from build123d import *

# Parameters (mm, degrees)
SKETCH1_R           = 2.2
SKETCH1_W           = 25.4
SKETCH1_H           = 25.4
SKETCH1_W_2         = 4.6228
SKETCH1_H_2         = 4.6228
SKETCH1_W_3         = 12.7
SKETCH1_H_3         = 12.7
BOSS_EXTRUDE1_DEPTH = 12.7
BOSS_EXTRUDE2_START = 12.7
SKETCH1_3_W         = 4.6228
SKETCH1_3_H         = 4.6228
BOSS_EXTRUDE2_DEPTH = 1.6
FILLET1_R           = 6.35
FILLET2_R           = 0.6
FILLET3_R           = 1


with BuildPart() as part:
    # Sketch1 → Boss-Extrude1 (new body)
    # profile 1 of 5: a face of its own
    with BuildSketch(Plane.XY):
        Polygon((6.35, -31.75), (0, -25.4), (25.4, -25.4), (25.4, 0), (31.75, -6.35), (44.45, -6.35), (44.45, -19.05), (76.2, -19.05), (76.2, -31.75), align=None)
        with Locations((38.1, -12.7)):
            Circle(SKETCH1_R, mode=Mode.SUBTRACT)
    # profile 2 of 5: a face of its own
    with BuildSketch(Plane.XY):
        with Locations((12.7, -12.7)):
            Rectangle(SKETCH1_W, SKETCH1_H)
        with Locations((19.05, -19.05)):
            Circle(SKETCH1_R, mode=Mode.SUBTRACT)
        with Locations((19.05, -6.35)):
            Circle(SKETCH1_R, mode=Mode.SUBTRACT)
        with Locations((6.35, -6.35)):
            Rectangle(SKETCH1_W_2, SKETCH1_H_2, mode=Mode.SUBTRACT)
        with Locations((6.35, -19.05)):
            Rectangle(SKETCH1_W_2, SKETCH1_H_2, mode=Mode.SUBTRACT)
    # profile 3 of 5: a face of its own
    with BuildSketch(Plane.XY):
        with Locations((6.35, -19.05)):
            Rectangle(SKETCH1_W_2, SKETCH1_H_2)
    # profile 4 of 5: a face of its own
    with BuildSketch(Plane.XY):
        with Locations((6.35, -6.35)):
            Rectangle(SKETCH1_W_2, SKETCH1_H_2)
    # profile 5 of 5: a face of its own
    with BuildSketch(Plane.XY):
        with Locations((82.55, -25.4)):
            Rectangle(SKETCH1_W_3, SKETCH1_H_3)
    extrude(amount=BOSS_EXTRUDE1_DEPTH)

    # Sketch1<3> → Boss-Extrude2 (add)
    with BuildSketch(Plane.XY.offset(BOSS_EXTRUDE2_START)):
        with Locations((6.35, -6.35)):
            Rectangle(SKETCH1_3_W, SKETCH1_3_H)
        with Locations((6.35, -19.05)):
            Rectangle(SKETCH1_3_W, SKETCH1_3_H)
    extrude(amount=BOSS_EXTRUDE2_DEPTH)

    # Fillet1
    fillet1_edges = [part.edges().sort_by_distance(p)[0] for p in [
        (88.9, -31.75, 6.35),
        (88.9, -19.05, 6.35),
        (44.45, -19.05, 6.35),
        (44.45, -6.35, 6.35),
        (31.75, -6.35, 6.35),
        (25.4, 0, 6.35),
        (6.35, -31.75, 6.35),
        (0, -25.4, 6.35),
        (0, 0, 6.35),
    ]]
    fillet(fillet1_edges, radius=FILLET1_R - 0.0001)  # a hair under: the kernel refuses the full size

    # Fillet2
    fillet2_edges = [part.edges().sort_by_distance(p)[0] for p in [
        (6.35, -8.6614, 14.3),
        (4.0386, -8.6614, 13.5),
        (8.6614, -8.6614, 13.5),
        (8.6614, -4.0386, 13.5),
        (4.0386, -6.35, 14.3),
        (4.0386, -4.0386, 13.5),
        (8.6614, -6.35, 14.3),
        (6.35, -4.0386, 14.3),
        (6.35, -21.3614, 14.3),
        (4.0386, -21.3614, 13.5),
        (8.6614, -21.3614, 13.5),
        (8.6614, -16.7386, 13.5),
        (4.0386, -19.05, 14.3),
        (4.0386, -16.7386, 13.5),
        (8.6614, -19.05, 14.3),
        (6.35, -16.7386, 14.3),
    ]]
    fillet(fillet2_edges, radius=FILLET2_R)

    # Fillet3
    fillet3_edges = [part.edges().sort_by_distance(p)[0] for p in [
        (3.175, -28.575, 0),
        (0, -14.55984265, 0),
        (14.55984265, 0, 0),
        (28.575, -3.175, 0),
        (36.24015735, -6.35, 0),
        (66.675, -19.05, 0),
        (45.76515735, -31.75, 0),
        (1.85984265, -1.85984265, 0),
        (0.483357357, -25.199786827, 0),
        (6.550213173, -31.266642643, 0),
        (25.199786827, -0.483357357, 0),
        (42.59015735, -8.20984265, 0),
        (87.04015735, -20.90984265, 0),
        (87.04015735, -29.89015735, 0),
        (45.76515735, -31.75, 12.7),
        (3.175, -28.575, 12.7),
        (66.675, -19.05, 12.7),
        (36.24015735, -6.35, 12.7),
        (28.575, -3.175, 12.7),
        (14.55984265, 0, 12.7),
        (0, -14.55984265, 12.7),
        (1.85984265, -1.85984265, 12.7),
        (0.483357357, -25.199786827, 12.7),
        (6.550213173, -31.266642643, 12.7),
        (25.199786827, -0.483357357, 12.7),
        (42.59015735, -8.20984265, 12.7),
        (87.04015735, -20.90984265, 12.7),
        (87.04015735, -29.89015735, 12.7),
        (46.30984265, -17.19015735, 0),
        (46.30984265, -17.19015735, 12.7),
        (31.950213173, -5.866642643, 0),
        (31.950213173, -5.866642643, 12.7),
    ]]
    fillet(fillet3_edges, radius=FILLET3_R)


solid = part.part
The listing builds one solid part. Answer for the finished solid, in the listing's coordinates (mm). A direction names the side the tool comes from. Give positions to 0.01 mm unless a question says otherwise; leave off trailing zeros. Write each loop counter-clockwise with the first axis right and the second up, starting at its lowest first coordinate (ties: lowest second). Pieces come first, ordered by that corner, then holes.
1) A tool of negligible diameter and unlimited length cuts with its end or side. For faces 4 (the face through (28.381, -3.406, 12.415)), 5 (the face through (66, -19.05, 6)), from which of +Z, -Z, +X, -X, +Y, -Y can it reach the whole face along a straight path? Write none if from no direction.
2) For a pull along Y with two mould halves and no side action, classify faces 1 (the face through (17.304, -20.389, 6.261)), 2 (the face through (1.91, -1.81, 6.42)), 3 (the face through (3.369, -28.344, 12.415)) as pulls with the +Y half, pulls with the -Y half, needs draft (parallel to the pull), parting line crosses it, or undercut.
3) Find the intervals of material crossed by L1, parallel to Y at x = 19.05, z = 4.5; L2, parallel to Y at x = 81.5, z = 3; L3, parallel to Z at x = 62, y = -26, in increasing order.
4) Given P1, Ø2, axis at x = 65, z = 5.5, coming from the +Y side; P2, Ø4, axis at x = 38.1, y = -12.7, coming from the -Z side; P3, Ø5, axis at x = 37, z = 9, coming from the +Y side; P4, Ø0.8, axis at x = 7, z = 13.5, coming from the +Y side, each flat-ended and moving along its own axis, determine where each tip first touches the part or whether it passes through.
5) Section A-A (z = 5) is taken. Count the separate pieces of the cut face and the enclosed holes in it, and give its area (3 significant figures).
6) Section C-C (x = 56.5) is taken. Write down the section's boundary in (y, z), and give its area (3 significant figures).
7) Section B-B (x = 19.05) is taken. Write down the section's boundary in (y, z), and give its area (3 significant figures).
Response:
1. face 4: +Z, +X, +Y
1. face 5: +Z, -Z, +X, +Y
2. face 1: undercut
2. face 2: pulls with the +Y half
2. face 3: pulls with the -Y half
3. L1: y = -31.75 to -21.25, -16.85 to -8.55, -4.15 to 0
3. L2: y = -31.75 to -19.05
3. L3: z = 0 to 12.7
4. P1: stops at y = -19.05
4. P2: passes through
4. P3: stops at y = -6.35
4. P4: stops at y = -4.04
5. separate pieces: 1
5. enclosed holes: 3
5. area: 1,780 mm2
6. outline: (-31.75, 1) arc R1 ccw to (-30.75, 0) - (-20.05, 0) arc R1 ccw to (-19.05, 1) - (-19.05, 11.7) arc R1 ccw to (-20.05, 12.7) - (-30.75, 12.7) arc R1 ccw to (-31.75, 11.7) - close
6. area: 160 mm2
7. outline: (-31.75, 1) arc R1 ccw to (-30.75, 0) - (-21.25, 0) - (-21.25, 12.7) - (-30.75, 12.7) arc R1 ccw to (-31.75, 11.7) - close; (-16.85, 0) - (-8.55, 0) - (-8.55, 12.7) - (-16.85, 12.7) - close; (-4.15, 0) - (-1, 0) arc R1 ccw to (0, 1) - (0, 11.7) arc R1 ccw to (-1, 12.7) - (-4.15, 12.7) - close
7. area: 291 mm2
